Check sheet for the modelled part. Datum: model origin and axes. Units: mm. Coordinates: 2 decimals unless noted, no trailing zeros. Write each loop counter-clockwise with the first axis right and the second up, starting at its lowest first coordinate (ties: lowest second). Pieces come first, ordered by that corner, then holes. Notation, with made-up numbers: (-2, 69.5) -> (17, 69.5) arc R28 cw to (17, 104.5) -> close; hole circle Ø3 at (-32.5, 17). An arc over 180 degrees is marked (long way). One line per item, written item: value. Start each with the question number.
1) Scan line: line 1 along X through (y, z) = (8, -18.5). Record every from-to range of solid material in increasing order. Write a range as [from, to].
2) Sectioned sample at A-A on z = -18. Enter the section's corners in (x, y).
3) Sectioned sample at B-B on y = 28.5. Enter the section's corners in (x, z).
4) Draft check along Y on faces 1 (the flat face through (-1, 32, 0)), 2 (the flat face through (-1, 16, -25)), 3 (the cylindrical face through (-84.084, 10.399, -24.908)), 4 (the flat face through (-1, 0, 0)). Enter one of: +Y half, -Y half, draft (parallel to the pull), parting line (faces both ways), or undercut.
```python
from build123d import *

# Parameters (mm, degrees)
SKETCH1_W           = 160
SKETCH1_H           = 50
BOSS_EXTRUDE1_DEPTH = 32
FILLET1_R           = 2
SKETCH2_R           = 2
BOSS_EXTRUDE2_DEPTH = 10


with BuildPart() as part:
    # Sketch1 → Boss-Extrude1 (new body)
    with BuildSketch(Plane(origin=(0, 0, 0), x_dir=(1, 0, 0), z_dir=(0, 1, 0))):
        Rectangle(SKETCH1_W, SKETCH1_H)
    extrude(amount=BOSS_EXTRUDE1_DEPTH)

    # Fillet1
    fillet1_edges = [part.edges().sort_by_distance(p)[0] for p in [
        (80, 32, 0),
        (0, 32, -25),
        (-80, 32, 0),
        (0, 0, -25),
        (80, 0, 0),
        (0, 0, 25),
        (-80, 0, 0),
        (0, 32, 25),
        (-80, 16, -25),
        (80, 16, -25),
        (80, 16, 25),
        (-80, 16, 25),
    ]]
    fillet(fillet1_edges, radius=FILLET1_R)

    # Sketch2 → Boss-Extrude2 (add, symmetric)
    with BuildSketch(Plane.ZY.offset(80)):
        with Locations(Location((-23, 21, 0), (0, 0, 180))):
            Circle(SKETCH2_R)
        with Locations(Location((-23, 16, 0), (0, 0, 180))):
            Circle(SKETCH2_R)
        with Locations(Location((-23, 11, 0), (0, 0, 180))):
            Circle(SKETCH2_R)
    extrude(amount=BOSS_EXTRUDE2_DEPTH, both=True)


solid = part.part
```
Answers:
1. line 1: x = [-80, 80]
2. outline: (-80, 2) arc R2 ccw to (-78, 0) -> (78, 0) arc R2 ccw to (80, 2) -> (80, 30) arc R2 ccw to (78, 32) -> (-78, 32) arc R2 ccw to (-80, 30) -> close
3. outline: (-80, -23) arc R2 ccw to (-78, -25) -> (78, -25) arc R2 ccw to (80, -23) -> (80, 23) arc R2 ccw to (78, 25) -> (-78, 25) arc R2 ccw to (-80, 23) -> close
4. face 1: +Y half
4. face 2: draft
4. face 3: undercut
4. face 4: -Y half
